The model under review builds one solid part; all positions refer to its coordinate system, in mm. Face numbers are marked on the shaded views. A direction names the side the tool comes from. Coordinates: 2 decimals unless noted, no trailing zeros. Loops run counter-clockwise (first coordinate to the right, second up) from the corner with the lowest first, then second, coordinate; pieces in that order, holes last. Notation, with made-up numbers: M 1.25,8 L 14.25,8 A12 cw 14.25,13 Z; hole C -13,23 d6. An arc over 180 degrees is marked long. One line per item, written item: value.
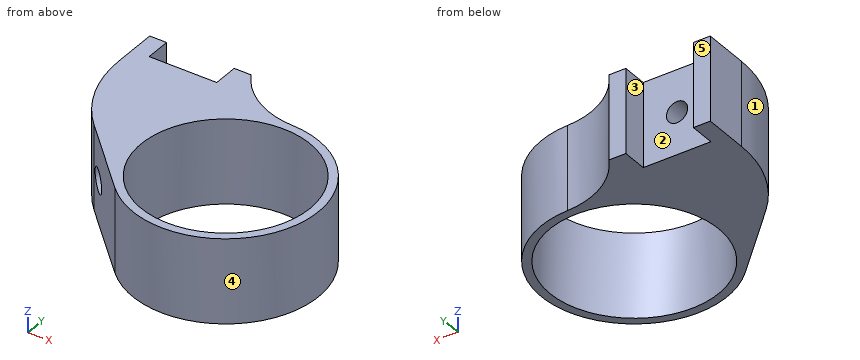
```python
from build123d import *

# Parameters (mm, degrees)
SKETCH1_R           = 10
BOSS_EXTRUDE1_DEPTH = 10
FILLET1_R           = 10
M3_TAPPED_HOLE1_D   = 2.5
FILLET2_R           = 15


with BuildPart() as part:
    # Sketch1 → Boss-Extrude1 (new body)
    with BuildSketch(Plane.XY):
        with BuildLine():
            Line((-18, 16), (-20, 16))
            Line((-20, 16), (-20, 4.443650814))
            Line((-20, 4.443650814), (-7.778174593, -7.778174593))
            ThreePointArc((-7.778174593, -7.778174593), (10.998848284, 0.159174228), (-8, 7.549834435))
            Line((-8, 7.549834435), (-8, 16))
            Line((-8, 16), (-10, 16))
            Line((-10, 16), (-10, 13))
            Line((-10, 13), (-18, 13))
            Line((-18, 13), (-18, 16))
        make_face()
        Circle(SKETCH1_R, mode=Mode.SUBTRACT)
    extrude(amount=BOSS_EXTRUDE1_DEPTH)

    # Fillet1
    # the kernel refuses this fillet: 10 mm, written as the material it adds along each edge
    with BuildSketch(Plane(origin=(-8, 7.549834435, 0), x_dir=(0, 1, 0), z_dir=(0, 0, 1))) as fillet1_piece_1:
        with BuildLine():
            CenterArc((13.43959092, -8.66635071), FILLET1_R, 119.930063337, 58.25157985)
            Line((3.444626465, -8.349040848), (3.244727176, -8.342694651))
            ThreePointArc((3.244727176, -8.342694651), (2.433829653, -3.880964752), (-0.137269717, -0.145454545))
            Line((-0.137269717, -0.145454545), (0, 0.2))
            ThreePointArc((0, 0.2), (4.225082782, 0.2), (8.350377058, 0.173327014))
            Line((8.350377058, 0.173327014), (8.450165565, 0))
        make_face()
    extrude(amount=10)

    # M3 Tapped Hole1 (through all)
    with Locations(Plane(origin=(0, 13, 0), x_dir=(1, 0, 0), z_dir=(0, 1, 0))):
        with Locations((-14, -5)):
            Hole(M3_TAPPED_HOLE1_D / 2)

    # Fillet2
    fillet2_edges = [part.edges().sort_by_distance(p)[0] for p in [
        (-20, 4.443650814, 5),
    ]]
    fillet(fillet2_edges, radius=FILLET2_R)


solid = part.part
```
(1) Insertion check: pin 1 Ø2 at (x, z) = (-5.5, 6) entering from -Y; pin 2 Ø3 at (x, z) = (-13.5, 3) entering from -Y; pin 3 Ø1.5 at (y, z) = (15, 3.5) entering from +X. Each pin has a flat end and moves straight along its axis. Give the tip position at first contact, or say it passes through.
Checks:
pin 1: y = -10.04
pin 2: y = -3.56
pin 3: x = -6.72
(2) Add section C-C on x = -2. State the section outline as (y, z) points.
Checks:
outline: M -10.82,0 L -9.8,0 L -9.8,10 L -10.82,10 Z; M 9.8,0 L 11.35,0 L 11.35,10 L 9.8,10 Z
(3) Add section D-D on z = 9.5. State the section outline as (x, y) points, then the cut area to 3 significant figures.
Checks:
outline: M -20,10.66 A15 ccw -15.61,0.05 L -7.78,-7.78 A11 ccw long 0.35,10.99 A10 cw -8,16 L -10,16 L -10,13 L -18,13 L -18,16 L -20,16 Z; hole C 0,0 d20
area: 238 mm^2
(4) To check wall thickness, follow L1, parallel to X at y = 5, z = 5; L2, parallel to X at y = 0.75, z = 5; L3, parallel to Z at x = -14, y = 3.75. State the ranges of each line that lie inside material, in increasing order. Write a range as [from, to].
Checks:
L1: [-18.89, -15.25], [-12.75, -8.66], [8.66, 9.8]
L2: [-16.26, -15.25], [-12.75, -9.97], [9.97, 10.97]
L3: [0, 3.75], [6.25, 10]
(5) Tool access review of the marked faces 1 and 2: name each direction out of +Z, -Z, +X, -X, +Y, -Y from which nothing blocks a thin tool from reaching the whole face with its end or side.
Checks:
face 1: +Z, -Z, -X, -Y
face 2: +Z, -Z, +Y
(6) Draft analysis for pull direction X (two halves, no side actions). For the marked faces 3, 4 and 5, state which applies: pulls with the +X half, pulls with the -X half, needs draft (parallel to the pull), parting line crosses it, or undercut.
Checks:
face 3: undercut
face 4: parting line crosses it
face 5: needs draft
(7) Add section B-B on z = 5. State the section outline as (x, y) points, then the cut area to 3 significant figures.
Checks:
outline: M -20,10.66 A15 ccw -15.61,0.05 L -15.25,-0.31 L -15.25,13 L -18,13 L -18,16 L -20,16 Z; M -12.75,-2.81 L -7.78,-7.78 A11 ccw long 0.35,10.99 A10 cw -8,16 L -10,16 L -10,13 L -12.75,13 Z; hole C 0,0 d20
area: 201 mm^2
(8) Add section A-A on y = 1.25. State the section outline as (x, z) points.
Checks:
outline: M -16.68,0 L -9.92,0 L -9.92,10 L -16.68,10 Z; M 9.92,0 L 10.93,0 L 10.93,10 L 9.92,10 Z; hole C -14,5 d2.5
